Geometry check sheet. Reference: the model listing, model coordinates, mm. A direction names the side the tool comes from. Round coordinates to 2 decimals unless told otherwise and drop trailing zeros. Order: outer loops, then holes, each group sorted by start corner. A loop starts at its lowest first (then second) coordinate and runs counter-clockwise, first axis right, second up. Notation, with made-up numbers: (-13.75, 0) - (18.25, 0) arc R16 cw to (18.25, 12) - close; hole circle Ø1 at (-27.75, 79). An arc over 180 degrees is marked (long way). Use a Markdown table: item, result. Add a question column.
(1) Thickness scan on line 1 along Y through (x, z) = (0, 0.2); line 2 along Z through (x, y) = (3.5, 3.5); line 3 along X through (y, z) = (0, 39.75). Record the ranges inside material, lowest first. Write a range as [from, to].
(2) Gauge pin test, flat ends, axial feed: P1, Ø3, axis at y = 0.5, z = 33, coming from the -X side; P2, Ø3, axis at x = 2, z = 35, coming from the -Y side. Record the tip position at first contact, or that the pin passes through.
(3) Section check D-D on z = 28.5. Record the boundary of the cut face in (x, y).
(4) Access from +Z, -Z, +X, -X, +Y, -Y to the whole of each face (thin tool, end or side, straight path). Record for faces 1 (the face through (5.3, 5.2, 36.1)), 2 (the face through (5.3, 5.2, 3.9)), 3 (the face through (5.3, -5.2, 36.1)).
(5) Section check C-C on x = -2.25. Record the boundary of the cut face in (y, z).
(6) Section check B-B on y = 0. Record the boundary of the cut face in (x, z), then the cut area to 3 significant figures.
(7) Section check A-A on x = 0. Record the boundary of the cut face in (y, z).
(8) Mould release check, pull along Z, two halves, no side actions. Record for faces 4 (the face through (2, 4, 39.6)), 5 (the face through (4, 2, 40)), 6 (the face through (4, 2, 0)), 7 (the face through (5.5, 0, 20)): released by +Z, released by -Z, zero draft, split by the parting line, or undercut.
```python
from build123d import *

# Parameters (mm, degrees)
SKETCH1_W           = 11
SKETCH1_H           = 12
BOSS_EXTRUDE1_DEPTH = 40
SKETCH2_W           = 10.6
SKETCH2_H           = 39.2
CUT_EXTRUDE1_DEPTH  = 43.121847063
CUT_EXTRUDE2_DEPTH  = 0.8
CHAMFER1_SIZE       = 0.8
CUT_EXTRUDE3_DEPTH  = 41.819725624
FILLET1_R           = 0.4


with BuildPart() as part:
    # Sketch1 → Boss-Extrude1 (new body)
    with BuildSketch(Plane.XY):
        Rectangle(SKETCH1_W, SKETCH1_H)
    extrude(amount=BOSS_EXTRUDE1_DEPTH)

    # Sketch2 → Cut-Extrude1 (cut, through all)
    with BuildSketch(Plane(origin=(0, 6, 0), x_dir=(1, 0, 0), z_dir=(0, 1, 0))):
        with Locations((-0.2, -20)):
            Rectangle(SKETCH2_W, SKETCH2_H)
    extrude(amount=-CUT_EXTRUDE1_DEPTH, mode=Mode.SUBTRACT)

    # Sketch3 → Cut-Extrude2 (cut)
    with BuildSketch(Plane(origin=(0, 6, 0), x_dir=(1, 0, 0), z_dir=(0, 1, 0))):
        Polygon((-5.5, 0), (5.5, 0), (5.5, -14.1), (5.1, -14.1), (5.1, -25.9), (5.5, -25.9), (5.5, -40), (-5.5, -40), align=None)
    cut_extrude2 = extrude(amount=-CUT_EXTRUDE2_DEPTH, mode=Mode.SUBTRACT)

    # Mirror1: Cut-Extrude2 across plane
    add(cut_extrude2.mirror(Plane.ZX), mode=Mode.SUBTRACT)

    # Chamfer1
    chamfer1_edges = [part.edges().sort_by_distance(p)[0] for p in [
        (5.3, -6, 25.9),
        (5.3, -6, 14.1),
        (5.3, 6, 25.9),
        (5.3, 6, 14.1),
    ]]
    chamfer(chamfer1_edges, length=CHAMFER1_SIZE - 0.0001)  # a hair under: the kernel refuses the full size

    # Sketch4 → Cut-Extrude3 (cut, through all)
    with BuildSketch(Plane(origin=(0, 0, 0), x_dir=(-1, 0, 0), z_dir=(0, 0, -1))):
        with BuildLine():
            Line((5.5, -3), (2.645751311, -3))
            ThreePointArc((2.645751311, -3), (-4, 0), (2.645751311, 3))
            Line((2.645751311, 3), (5.5, 3))
            Line((5.5, 3), (5.5, -3))
        make_face()
    extrude(amount=-CUT_EXTRUDE3_DEPTH, mode=Mode.SUBTRACT)

    # Fillet1
    fillet1_edges = [part.edges().sort_by_distance(p)[0] for p in [
        (-5.5, 3, 0.2),
        (-5.5, 3, 39.8),
        (-5.5, -3, 0.2),
        (-5.5, -3, 39.8),
        (-5.5, 5.2, 0.2),
        (-5.5, 5.2, 39.8),
        (-5.5, -5.2, 39.8),
        (-5.5, -5.2, 0.2),
    ]]
    fillet(fillet1_edges, radius=FILLET1_R)


solid = part.part
```
Check sheet entries:
| question | item | result |
|---|---|---|
| 1 | line 1 | y = [-5.2, -4], [4, 5.2] |
| 1 | line 2 | z = [0, 0.4], [39.6, 40] |
| 1 | line 3 | x = [4, 5.5] |
| 2 | P1 | stops at x = 5.1 |
| 2 | P2 | passes through |
| 3 | outline | (5.1, -5.2) - (5.5, -5.2) - (5.5, 5.2) - (5.1, 5.2) - close |
| 4 | face 1 | +Z, +X, -X, +Y |
| 4 | face 2 | -Z, +X, -X, +Y |
| 4 | face 3 | +Z, +X, -X, -Y |
| 5 | outline | (-5.2, 0) - (-3.31, 0) - (-3.31, 0.4) - (-5.2, 0.4) - close; (-5.2, 39.6) - (-3.31, 39.6) - (-3.31, 40) - (-5.2, 40) - close; (3.31, 0) - (5.2, 0) - (5.2, 0.4) - (3.31, 0.4) - close; (3.31, 39.6) - (5.2, 39.6) - (5.2, 40) - (3.31, 40) - close |
| 6 | outline | (4, 0) - (5.5, 0) - (5.5, 40) - (4, 40) - (4, 39.6) - (5.1, 39.6) - (5.1, 0.4) - (4, 0.4) - close |
| 6 | area | 16.9 mm2 |
| 7 | outline | (-5.2, 0) - (-4, 0) - (-4, 0.4) - (-5.2, 0.4) - close; (-5.2, 39.6) - (-4, 39.6) - (-4, 40) - (-5.2, 40) - close; (4, 0) - (5.2, 0) - (5.2, 0.4) - (4, 0.4) - close; (4, 39.6) - (5.2, 39.6) - (5.2, 40) - (4, 40) - close |
| 8 | face 4 | undercut |
| 8 | face 5 | released by +Z |
| 8 | face 6 | released by -Z |
| 8 | face 7 | zero draft |
